from build123d import *

# Parameters (mm, degrees)
F0_W     = 119.0162692178
F0_H     = 19.05
F1_DEPTH = 63.5
F2_W     = 118.98781716
F2_H     = 50.8
F3_DEPTH = 19.05
F5_DEPTH = 25.4
F6_R     = 19.05
F7_R     = 19.05


with BuildPart() as f1:
    # F0 (on Front) → F1 (new body)
    with BuildSketch(Plane.XZ):
        with Locations((-0.0617158565, 9.525)):
            Rectangle(F0_W, F0_H)
    extrude(amount=F1_DEPTH)

    # F2 (on Front) → F3 (join)
    with BuildSketch(Plane.XZ):
        with Locations((0.0594016165, 44.4325357676)):
            Rectangle(F2_W, F2_H)
    extrude(amount=F3_DEPTH)

    # F4 (on face) → F5 (cut)
    with BuildSketch(Plane.XY.offset(19.05)):
        with BuildLine():
            Line((-12.7617158565, -63.5), (12.6382841435, -63.5))
            ThreePointArc((12.6382841435, -63.5), (-0.0617158565, -50.8), (-12.7617158565, -63.5))
        make_face()
    extrude(amount=-F5_DEPTH, mode=Mode.SUBTRACT)

    # F6
    f6_edges = [f1.edges().sort_by_distance(p)[0] for p in [
        (-59.434507, -9.525, 69.832536),
    ]]
    fillet(f6_edges, radius=F6_R)

    # F7
    f7_edges = [f1.edges().sort_by_distance(p)[0] for p in [
        (59.55331, -9.525, 69.832536),
    ]]
    fillet(f7_edges, radius=F7_R)


solid = f1.part
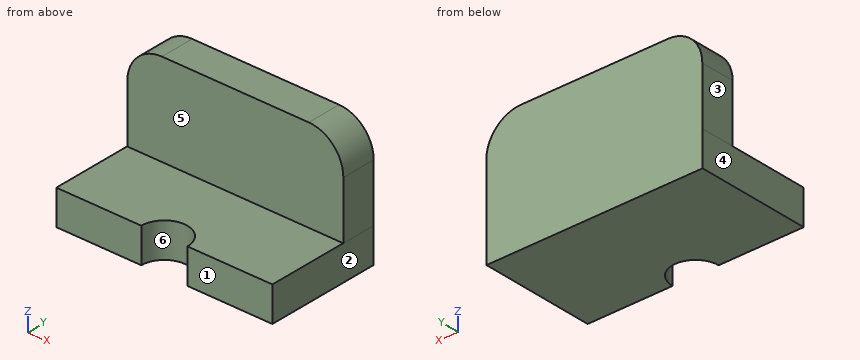
Geometry check sheet. Reference: the model listing, model coordinates, mm. Face numbers are marked on the shaded views. A direction names the side the tool comes from. Coordinates: 2 decimals unless noted, no trailing zeros. Order: outer loops, then holes, each group sorted by start corner. A loop starts at its lowest first (then second) coordinate and runs counter-clockwise, first axis right, second up. Notation, with made-up numbers: (6.25, -0.5) -> (47.25, -0.5) arc R30 ccw to (47.25, 31.5) -> close; hole circle Ø10 at (77, 5). An arc over 180 degrees is marked (long way). Use a Markdown table: item, result. Add a question column.
1. Mould release check, pull along X, two halves, no side actions. Record for the marked faces 4, 5 and 6: pulls with the +X half, pulls with the -X half, needs draft (parallel to the pull), parting line crosses it, or undercut.
2. Set-up check for the marked faces 1, 2 and 3: record each of +Z, -Z, +X, -X, +Y, -Y from which the full face is reachable in a straight line by a thin tool's end or side.
3. Cross-section at B-B (y = -55). Enter the section's corners in (x, z).
4. Cross-section at C-C (z = 11). Enter the section's corners in (x, y).
5. Cross-section at A-A (x = 17.5). Enter the section's corners in (y, z), and give its area (3 significant figures).
6. Go/stop test with flat-tipped pins: pin 1 Ø12 at (y, z) = (-28, 13) entering from +X; pin 2 Ø9.5 at (y, z) = (-12.5, 37) entering from -X; pin 3 Ø12 at (x, z) = (-1, 52) entering from -Y. Record where each tip stops, or that it passes through.
7. Cross-section at D-D (y = -17). Enter the section's corners in (x, z), and give its area (3 significant figures).
8. Material ranges on L1, parallel to Y at x = -32, z = 55; L2, parallel to Z at x = -17, y = -36; L3, parallel to X at y = -31, z = 15, recorded low to high.
Filled sheet:
| question | item | result |
|---|---|---|
| 1 | face 4 | pulls with the -X half |
| 1 | face 5 | needs draft |
| 1 | face 6 | undercut |
| 2 | face 1 | +Z, -Z, +X, -X, -Y |
| 2 | face 2 | -Z, +X, +Y, -Y |
| 2 | face 3 | +Z, -X, +Y, -Y |
| 3 | outline | (-59.57, 0) -> (-9.5, 0) -> (-9.5, 19.05) -> (-59.57, 19.05) -> close; (9.37, 0) -> (59.45, 0) -> (59.45, 19.05) -> (9.37, 19.05) -> close |
| 4 | outline | (-59.57, -63.5) -> (-12.76, -63.5) arc R12.7 cw to (12.64, -63.5) -> (59.45, -63.5) -> (59.45, 0) -> (-59.57, 0) -> close |
| 5 | outline | (-63.5, 0) -> (0, 0) -> (0, 69.83) -> (-19.05, 69.83) -> (-19.05, 19.05) -> (-63.5, 19.05) -> close |
| 5 | area | 2,180 mm2 |
| 6 | pin 1 | x = 59.45 |
| 6 | pin 2 | x = -59.43 |
| 6 | pin 3 | y = -19.05 |
| 7 | outline | (-59.57, 0) -> (59.45, 0) -> (59.45, 19.03) -> (59.55, 19.03) -> (59.55, 50.78) arc R19.05 ccw to (40.5, 69.83) -> (-40.38, 69.83) arc R19.05 ccw to (-59.43, 50.78) -> (-59.43, 19.05) -> (-59.57, 19.05) -> close |
| 7 | area | 8,150 mm2 |
| 8 | L1 | -19.05 to 0 |
| 8 | L2 | 0 to 19.05 |
| 8 | L3 | -59.57 to 59.45 |
